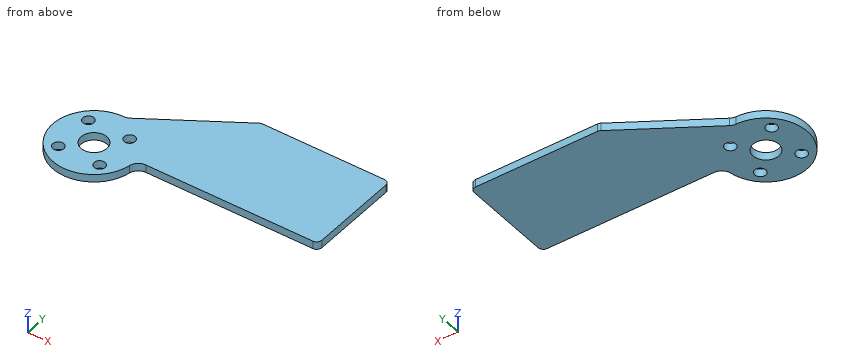
from build123d import *

# Parameters (mm, degrees)
SKETCH_R   = 2.15
SKETCH_R_2 = 5
PAD_DEPTH  = 3


with BuildPart() as part:
    # Sketch → Pad (new body)
    with BuildSketch(Plane.XY):
        with BuildLine():
            Line((36.7, 0.5), (84.5, 0.5))
            ThreePointArc((84.5, 0.5), (85.914214, 1.085786), (86.5, 2.5))
            Line((86.5, 2.5), (86.5, 36.6))
            ThreePointArc((86.5, 36.6), (85.914214, 38.014214), (84.5, 38.6))
            Line((84.5, 38.6), (37.282104, 38.6))
            ThreePointArc((37.282104, 38.6), (36.723192, 38.520317), (36.208816, 38.287617))
            Line((2.146577, 16.624765), (36.208816, 38.287617))
            ThreePointArc((0, 16), (1.117824, 16.159366), (2.146577, 16.624765))
            ThreePointArc((0, 16), (-12.263768, -10.276186), (15.753095, -2.8))
            ThreePointArc((19.691369, 0.5), (17.122322, -0.434058), (15.753095, -2.8))
            Line((36.7, 0.5), (19.691369, 0.5))
        make_face()
        with Locations((-8, 8)):
            Circle(SKETCH_R, mode=Mode.SUBTRACT)
        with Locations((8, 8)):
            Circle(SKETCH_R, mode=Mode.SUBTRACT)
        with Locations((-8, -8)):
            Circle(SKETCH_R, mode=Mode.SUBTRACT)
        with Locations((8, -8)):
            Circle(SKETCH_R, mode=Mode.SUBTRACT)
        Circle(SKETCH_R_2, mode=Mode.SUBTRACT)
    extrude(amount=PAD_DEPTH)


solid = part.part
Input: part model. Units: mm. Frame: model coordinates. Coordinates: 2 decimals unless noted, no trailing zeros. Loops run counter-clockwise (first coordinate to the right, second up) from the corner with the lowest first, then second, coordinate; pieces in that order, holes last.
Q1. Cut plane B-B (y = -8). Output: boundary loops of the cut face in (x, z).
Q2. Cut plane C-C (x = 8). Output: boundary loops of the cut face in (y, z).
Q3. Cut plane D-D (y = 33). Output: boundary loops of the cut face in (x, z).
Q4. Contact query for flat-ended pins moving along their axis: pin 1 (1 mm diameter, centred on x = 31, z = 2.5, fed in from -Y); pin 2 (10 mm diameter, centred on x = 25, y = -7.5, fed in from -Z). Output: stop coordinate, or through.
Q5. Cut plane A-A (z = 1.95). Output: boundary loops of the cut face in (x, y).
Q6. Material intervals for line 1 (Y direction, x = -8, z = 1.55); line 2 (X direction, y = 3.5, z = 1.4); line 3 (Y direction, x = -9, z = 2.8), sorted ascending.
Working result:
1. outline: (-13.86, 0) - (-10.15, 0) - (-10.15, 3) - (-13.86, 3) - close; (-5.85, 0) - (5.85, 0) - (5.85, 3) - (-5.85, 3) - close; (10.15, 0) - (13.86, 0) - (13.86, 3) - (10.15, 3) - close
2. outline: (-13.86, 0) - (-10.15, 0) - (-10.15, 3) - (-13.86, 3) - close; (-5.85, 0) - (5.85, 0) - (5.85, 3) - (-5.85, 3) - close; (10.15, 0) - (20.35, 0) - (20.35, 3) - (10.15, 3) - close
3. outline: (27.89, 0) - (86.5, 0) - (86.5, 3) - (27.89, 3) - close
4. pin 1: stops at y = 0.5
4. pin 2: passes through
5. outline: (0, 16) arc R16 ccw (long way) to (15.75, -2.8) arc R4 cw to (19.69, 0.5) - (84.5, 0.5) arc R2 ccw to (86.5, 2.5) - (86.5, 36.6) arc R2 ccw to (84.5, 38.6) - (37.28, 38.6) arc R2 ccw to (36.21, 38.29) - (2.15, 16.62) arc R4 cw to start; hole circle Ø4.3 at (-8, -8); hole circle Ø4.3 at (-8, 8); hole circle Ø10 at (0, 0); hole circle Ø4.3 at (8, -8); hole circle Ø4.3 at (8, 8)
6. line 1: y = -13.86 to -10.15, -5.85 to 5.85, 10.15 to 13.86
6. line 2: x = -15.61 to -3.57, 3.57 to 86.5
6. line 3: y = -13.23 to -9.9, -6.1 to 6.1, 9.9 to 13.23
